Here's how the part is built. I have some questions about the finished solid (model axes, mm). Face numbers are marked on the shaded views. A direction names the side the tool comes from. Give positions to 0.01 mm unless a question says otherwise; leave off trailing zeros. Order: outer loops, then holes, each group sorted by start corner. A loop starts at its lowest first (then second) coordinate and runs counter-clockwise, first axis right, second up. Notation, with made-up numbers: (72.5, 2.5) -> (96.5, 2.5) arc R22 ccw to (96.5, 17.5) -> close; hole circle Ø8 at (-34.75, 77.5). An arc over 180 degrees is marked (long way). Write each question's results on one line, items separated by ' | '. Start each with the question number.
Q1. I need wall thicknesses on line 1 along Y through (x, z) = (0.15, 0); line 2 along X through (y, z) = (-11, 6.25); line 3 along Y through (x, z) = (59, 8.75). Which ranges of each line are inside material? Lowest first, please. Write a range as [from, to].
Q2. For the marked faces 1 and 2, which set-ups out of +Z, -Z, +X, -X, +Y, -Y let a thin tool reach every point of the face, with its end or its side?
Q3. Imagine slicing it at C-C, the plane y = -41. Please give me the cut outline in (x, z) (1 decimal).
Q4. Imagine slicing it at A-A, the plane y = -19.05. Please give me the cut outline in (x, z), then the cut area to 3 significant figures.
Q5. Imagine slicing it at B-B, the plane x = 54. Please give me the cut outline in (y, z) (3 decimals), then the cut area to 3 significant figures.
Q6. I'm going to push flat-ended pins straight in: pin 1 (5 mm diameter, centred on x = 32.5, z = 3.5, fed in from -Y); pin 2 (1 mm diameter, centred on y = -29.5, z = -4, fed in from +X); pin 3 (4 mm diameter, centred on y = -6.35, z = 0, fed in from -X). Where does each tip first touch, or does it pass through?
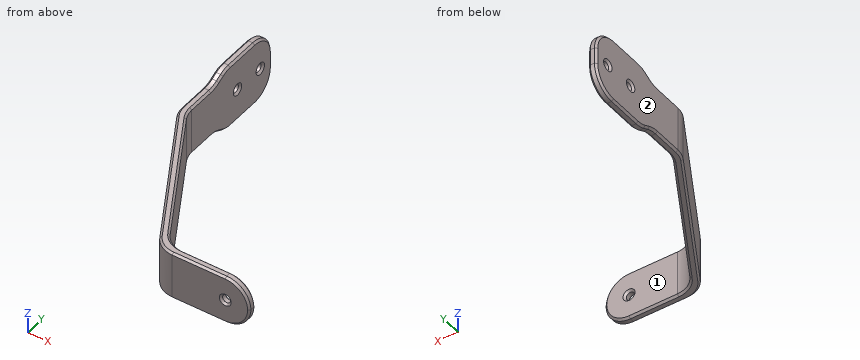
```python
from build123d import *

# Parameters (mm, degrees)
SKETCH2_W               = 3.175
SKETCH2_H               = 19.05
BOSS_EXTRUDE1_DEPTH     = 1.5875
CUT_EXTRUDE1_DEPTH      = 128.966941084
CUT_EXTRUDE1_DEPTH_BACK = 128.966941084
SKETCH8_R               = 1.5875
CUT_EXTRUDE2_DEPTH      = 126.316205076
CUT_EXTRUDE2_DEPTH_BACK = 126.316205076
SKETCH9_R               = 1.5875
FILLET1_R               = 9.525
CHAMFER1_SIZE           = 0.762


with BuildPart() as part:
    # Sweep1: sweep along a path in Sketch1
    with BuildLine(Plane.XY) as sweep1_path:
        Line((0, 0), (0, -47.5145354))
        Line((0, -47.5145354), (33.61082832, -105.730197734))
        Line((33.61082832, -105.730197734), (68.53582832, -105.730197734))
    # Sketch2 → Sweep1 (sweep)
    with BuildSketch(Plane(origin=(0, 0, 0), x_dir=(1, 0, 0), z_dir=(0, 1, 0))):
        Rectangle(SKETCH2_W, SKETCH2_H)
    sweep(path=sweep1_path.line, transition=Transition.RIGHT)

    # Sketch7 → Boss-Extrude1 (add, symmetric)
    with BuildSketch(Plane(origin=(0, 0, 0), x_dir=(0, 0, -1), z_dir=(1, 0, 0))):
        Polygon((-12.7, -25.4), (-9.525, -31.75), (9.525, -31.75), (12.7, -25.4), (12.7, 0), (-12.7, 0), align=None)
    extrude(amount=BOSS_EXTRUDE1_DEPTH, both=True)

    # Sketch8 → Cut-Extrude1 (cut, two sides: drawn at the far end of the back side and taken through both)
    with BuildSketch(Plane(origin=(0, 0, 0), x_dir=(0, 0, -1), z_dir=(1, 0, 0)).offset(-CUT_EXTRUDE1_DEPTH_BACK)):
        with Locations((0, -6.35)):
            Circle(SKETCH8_R)
        with Locations((0, -19.05)):
            Circle(SKETCH8_R)
    extrude(amount=CUT_EXTRUDE1_DEPTH + CUT_EXTRUDE1_DEPTH_BACK, mode=Mode.SUBTRACT)

    # Sketch9 → Cut-Extrude2 (cut, two sides: drawn at the far end of the back side and taken through both)
    with BuildSketch(Plane(origin=(0, -104.142697734, 0), x_dir=(1, 0, 0), z_dir=(0, 1, 0)).offset(-CUT_EXTRUDE2_DEPTH_BACK)):
        with Locations(Location((59.01082832, 0, 0), (0, 0, 180))):
            Circle(SKETCH9_R)
    extrude(amount=CUT_EXTRUDE2_DEPTH + CUT_EXTRUDE2_DEPTH_BACK, mode=Mode.SUBTRACT)

    # Fillet1
    fillet1_edges = [part.edges().sort_by_distance(p)[0] for p in [
        (0, -31.75, -9.525),
        (0, -25.4, -12.7),
        (0, -31.75, 9.525),
        (0, -25.4, 12.7),
        (0, 0, -12.7),
        (0, 0, 12.7),
        (68.53582832, -105.730197734, -9.525),
        (68.53582832, -105.730197734, 9.525),
        (1.5875, -47.089166057, 0),
        (-1.5875, -47.939904743, 0),
        (32.694284767, -107.317697734, 0),
        (34.527371872, -104.142697734, 0),
    ]]
    fillet(fillet1_edges, radius=FILLET1_R - 0.0001)  # a hair under: the kernel refuses the full size

    # Chamfer1
    chamfer1_edges = [part.edges().sort_by_distance(p)[0] for p in [
        (14.816638805, -76.352706607, 9.525),
        (14.816638805, -76.352706607, -9.525),
        (33.431038346, -106.041603103, -9.525),
        (-1.262946903, -47.852941003, -9.525),
        (-1.5875, -39.693119679, -9.525),
        (-1.262946903, -47.852941003, -9.525),
        (-1.5875, 0, 0),
        (-1.5875, -16.338188061, -12.7),
        (-1.5875, -28.575, -11.1125),
        (-1.5875, -39.693119679, 9.525),
        (-1.5875, -28.575, 11.1125),
        (-1.5875, -16.338188061, 12.7),
        (-1.5875, -2.78977862, 9.91022138),
        (-1.5875, -2.78977862, -9.91022138),
        (-1.5875, -25.339849714, 12.4451993),
        (-1.5875, -25.339849714, -12.4451993),
        (-1.262946903, -47.852941003, 9.525),
        (33.431038346, -106.041603103, 9.525),
        (-1.262946903, -47.852941003, 9.525),
        (48.602208333, -107.317697734, -9.525),
        (48.602208333, -107.317697734, 9.525),
        (65.7460497, -107.317697734, 6.73522138),
        (65.7460497, -107.317697734, -6.73522138),
        (49.518751885, -104.142697734, -9.525),
        (33.431038346, -106.041603103, -9.525),
        (49.518751885, -104.142697734, 9.525),
        (33.431038346, -106.041603103, 9.525),
        (65.7460497, -104.142697734, 6.73522138),
        (65.7460497, -104.142697734, -6.73522138),
        (1.912053097, -47.002202317, 9.525),
        (1.912053097, -47.002202317, 9.525),
        (1.912053097, -47.002202317, -9.525),
        (1.912053097, -47.002202317, -9.525),
        (35.264125451, -102.866603103, 9.525),
        (35.264125451, -102.866603103, 9.525),
        (35.264125451, -102.866603103, -9.525),
        (35.264125451, -102.866603103, -9.525),
        (-1.5875, -31.810150286, -9.7798007),
        (1.5875, -31.810150286, -9.7798007),
        (-1.5875, -31.810150286, 9.7798007),
        (1.5875, -31.810150286, 9.7798007),
        (-1.5875, -6.35, 1.5875),
        (1.5875, -6.35, 1.5875),
        (-1.5875, -19.05, 1.5875),
        (1.5875, -19.05, 1.5875),
        (60.59832832, -107.317697734, 0),
        (60.59832832, -104.142697734, 0),
        (17.320682357, -74.339837264, -9.525),
        (17.320682357, -74.339837264, 9.525),
        (1.5875, 0, 0),
        (1.5875, -16.338188061, 12.7),
        (1.5875, -28.575, 11.1125),
        (1.5875, -39.267750336, 9.525),
        (1.5875, -39.267750336, -9.525),
        (1.5875, -28.575, -11.1125),
        (1.5875, -16.338188061, -12.7),
        (1.5875, -2.78977862, 9.91022138),
        (1.5875, -2.78977862, -9.91022138),
        (1.5875, -25.339849714, 12.4451993),
        (1.5875, -25.339849714, -12.4451993),
    ]]
    chamfer(chamfer1_edges, length=CHAMFER1_SIZE)


solid = part.part
```
Geometry check:
1) line 1: [-50.95, -20.64], [-17.46, -7.94], [-4.76, 0] | line 2: [-1.59, 1.59] | line 3: [-107.32, -104.14]
2) face 1: +Z, -Z, +X, +Y | face 2: +Z, -Z, -X, +Y, -Y
3) outline: (-1.6, -8.8) -> (-0.8, -9.5) -> (0.8, -9.5) -> (1.6, -8.8) -> (1.6, 8.8) -> (0.8, 9.5) -> (-0.8, 9.5) -> (-1.6, 8.8) -> close
4) outline: (-1.59, -11.94) -> (-0.83, -12.7) -> (0.83, -12.7) -> (1.59, -11.94) -> (1.59, -2.35) -> (0.83, -1.59) -> (-0.83, -1.59) -> (-1.59, -2.35) -> close; (-1.59, 2.35) -> (-0.83, 1.59) -> (0.83, 1.59) -> (1.59, 2.35) -> (1.59, 11.94) -> (0.83, 12.7) -> (-0.83, 12.7) -> (-1.59, 11.94) -> close | area: 68.2 mm²
5) outline: (-107.318, -8.763) -> (-106.556, -9.525) -> (-104.905, -9.525) -> (-104.143, -8.763) -> (-104.143, 8.763) -> (-104.905, 9.525) -> (-106.556, 9.525) -> (-107.318, 8.763) -> close | area: 59.3 mm²
6) pin 1: y = -106.77 | pin 2: x = 1.59 | pin 3: x = -1.24
